The listing builds one solid part. Answer for the finished solid, in the listing's coordinates (mm). Face numbers are marked on the shaded views. A direction names the side the tool comes from. Round coordinates to 2 decimals unless told otherwise and drop trailing zeros. Loops run counter-clockwise (first coordinate to the right, second up) from the corner with the lowest first, then second, coordinate; pieces in that order, holes last. Notation, with made-up numbers: (77, 11) - (121, 11) arc R24 ccw to (121, 45) - close; hole circle Ø5 at (-36.75, 40). An arc over 180 degrees is marked (long way). One line per item, written item: value.
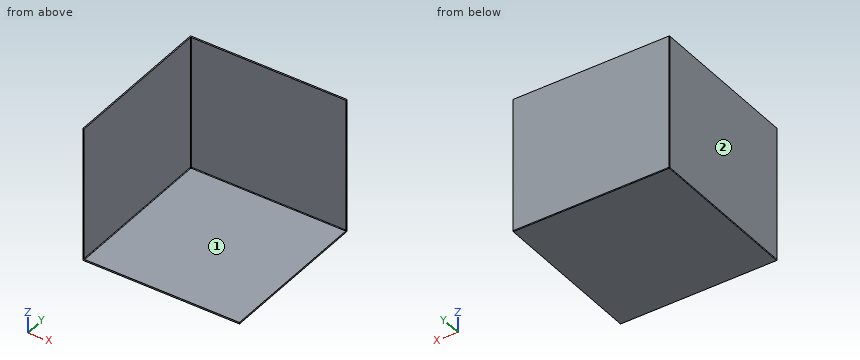
```python
from build123d import *

# Parameters (mm, degrees)
F0_W     = 5
F0_H     = 430
F1_DEPTH = 500
F2_W     = 500
F2_H     = 500
F3_DEPTH = 5
F4_W     = 4
F4_H     = 495
F5_DEPTH = 430
F7_R     = 2


# Not quite as in the source:
# - a feature names something its author has since deleted; it is built from what else it names


with BuildPart() as f1:
    # F0 (on Right) → F1 (new body)
    with BuildSketch(Plane.YZ):
        with Locations((-2.5, 215)):
            Rectangle(F0_W, F0_H)
    extrude(amount=F1_DEPTH)

    # F2 (on Top) → F3 (join)
    with BuildSketch(Plane.XY):
        with Locations((250, -250)):
            Rectangle(F2_W, F2_H)
    extrude(amount=F3_DEPTH)


with BuildPart() as f5:
    # F4 (on face) → F5 (new body, through all)
    with BuildSketch(Plane.XY.offset(430)):
        with Locations((2, -252.5)):
            Rectangle(F4_W, F4_H)
    extrude(amount=-F5_DEPTH)

    # F6: union F1
    add(f1.part)

    # F7
    f7_edges = [f5.edges().sort_by_distance(p)[0] for p in [
        (0, 0, 215),
        (250, 0, 0),
        (0, -250, 0),
        (252, -5, 5),
        (4, -5, 217.5),
        (4, -252.5, 5),
    ]]
    fillet(f7_edges, radius=F7_R)


solid = f5.part
```
1) Each of these flat-tipped pins is pushed along its axis until it touches: pin 1 Ø6 at (x, y) = (390, -85.5) entering from +Z; pin 2 Ø1.5 at (x, z) = (106.5, 280.5) entering from -Y. Where does it stop, or does it pass through?
Final values:
pin 1: z = 5
pin 2: y = -5
2) A cutting plane is placed at B-B on z = 229.5. Give the vertices of the cut face in (x, y).
Final values:
outline: (0, -500) - (4, -500) - (4, -7) arc R2 cw to (6, -5) - (500, -5) - (500, 0) - (2, 0) arc R2 ccw to (0, -2) - close
3) A cutting plane is placed at A-A on y = -402. Give the vertices of the cut face in (x, z), and give its area (3 significant figures).
Final values:
outline: (0, 2) arc R2 ccw to (2, 0) - (500, 0) - (500, 5) - (6, 5) arc R2 cw to (4, 7) - (4, 430) - (0, 430) - close
area: 4,200 mm2
4) Consider L1, parallel to Y at x = 152.5, z = 326.5; L2, parallel to X at y = -410, z = 291; L3, parallel to Z at x = 34.5, y = -130.5. Determine where each line is inside the solid, lowest interval first.
Final values:
L1: -5 to 0
L2: 0 to 4
L3: 0 to 5
5) For the marked faces 1 and 2, determine the directions among +Z, -Z, +X, -X, +Y, -Y from which every point of the face is accessible in a straight line to the end or side of a thin tool.
Final values:
face 1: +Z, +X, -Y
face 2: +Z, -Z, -X, +Y, -Y
